Autodesk Inventor part; units mm, degrees
ref_plane "YZ Plane" through (0, 0, 0) normal (1, 0, 0) x (0, 1, 0)
ref_plane "XZ Plane" through (0, 0, 0) normal (0, 1, 0) x (-1, 0, 0)
ref_plane "XY Plane" through (0, 0, 0) normal (0, 0, 1) x (1, 0, 0)
sketch "Boceto1" plane through (0, 0, 0) normal (0, 0, 1) x (1, 0, 0)
  line L0 (0, 0) -> (11.3785, 0)
  line L1 (0, 5) -> (10, 5)
  line L2 (10, 5) -> (10, 14)
  line L3 (10, 14) -> (5, 14)
  line L4 (5, 14) -> (5, 7.5)
  line L5 (5, 7.5) -> (0, 7.5)
  line L6 (0, 7.5) -> (0, 5)
  dimension "d0" = 5
  dimension "d1" = 5
  dimension "d3" = 28
  dimension "d4" = 15
  dimension "d5" = 10
revolve "Revolución1" add sketch "Boceto1" angle 360 about axis through (0, 0, 0) along (1, 0, 0)
fillet "Empalme1" radius 1 1 edges at (5, -7.5, 0)
chamfer "Chaflán1" distance 1 angle 45 1 edges at (5, -14, 0)
sketch "Boceto2" plane through (10, 0, 0) normal (1, 0, 0) x (0, 0, -1)
  circle A0 centre (0, 0) radius 14
  line L0 (-12, 12) -> (12, 12)
  line L1 (12, 12) -> (12, -12)
  line L2 (12, -12) -> (-12, -12)
  line L3 (-12, -12) -> (-12, 12)
  point P0 (12, 0)
  point P1 (0, 12)
  point P2 (-7.2111, 12)
  point P3 (7.2111, 12)
  point P4 (12, 7.2111)
  point P5 (12, -7.2111)
  point P6 (-12, -7.2111)
  point P7 (-12, 7.2111)
  point P8 (7.2111, -12)
  point P9 (-7.2111, -12)
  dimension "d11" = 24
  dimension "d12" = 24
extrude "Extrusión1" cut sketch "Boceto2" against normal blind 2.5 contours A0 L1 | L0 A0 | A0 L2 | L3 A0
thread "Rosca1"
properties part number "tuerca_manzana_1"
Can you work these out from the model? Positions are in its coordinate system, mm. A direction names the side the tool comes from. Coordinates: 2 decimals unless noted, no trailing zeros. Loops run counter-clockwise (first coordinate to the right, second up) from the corner with the lowest first, then second, coordinate; pieces in that order, holes last. Notation, with made-up numbers: (28.25, 31.25) -> (39.25, 31.25) arc R30 ccw to (39.25, 58.25) -> close; hole circle Ø2 at (12.25, -12.75). An arc over 180 degrees is marked (long way). Answer as a JSON object with one key per item and string values.
1) Imagine slicing it at D-D (x = 1.5). Please give me the cut outline in (y, z).
Results:
{"outline": "circle Ø15 at (0, 0); hole circle Ø10 at (0, 0)"}
2) Imagine slicing it at A-A (y = 0). Please give me the cut outline in (x, z), then the cut area to 3 significant figures.
Results:
{"outline": "(0, -7.5) -> (4, -7.5) arc R1 cw to (5, -8.5) -> (5, -13) -> (6, -14) -> (7.5, -14) -> (7.5, -12) -> (10, -12) -> (10, -5) -> (0, -5) -> close; (0, 5) -> (10, 5) -> (10, 12) -> (7.5, 12) -> (7.5, 14) -> (6, 14) -> (5, 13) -> (5, 8.5) arc R1 cw to (4, 7.5) -> (0, 7.5) -> close", "area": "104 mm^2"}
3) Imagine slicing it at C-C (x = 8.25). Please give me the cut outline in (y, z).
Results:
{"outline": "(-12, -7.21) arc R14 ccw to (-7.21, -12) -> (7.21, -12) arc R14 ccw to (12, -7.21) -> (12, 7.21) arc R14 ccw to (7.21, 12) -> (-7.21, 12) arc R14 ccw to (-12, 7.21) -> close; hole circle Ø10 at (0, 0)"}
4) For faces 1 (the face through (9, 12, 0)), 2 (the face through (9, -12, 0)), 3 (the face through (1.972, -7.493, -0.33)), which set-ups out of +Z, -Z, +X, -X, +Y, -Y let a thin tool reach every point of the face, with its end or its side?
Results:
{"face 1": "+Z, -Z, +X, +Y", "face 2": "+Z, -Z, +X, -Y", "face 3": "-X"}
5) If I drill on line 1 (Z direction, x = 6.75, y = 0); line 2 (Z direction, x = 2, y = 0); line 3 (X direction, y = 5.75, z = -10), over which ranges is the centre line in solid material (lowest first)?
Results:
{"line 1": "z = -14 to -5, 5 to 14", "line 2": "z = -7.5 to -5, 5 to 7.5", "line 3": "x = 5 to 10"}
6) For P1, Ø5, axis at x = 3.5, y = 2.5, coming from the +Z side; P2, Ø3, axis at x = 9.5, y = -0.5, coming from the +Z side; P3, Ø2, axis at y = 13.5, z = -1.5, coming from the +X side; P4, Ø3, axis at y = 2.5, z = 0.5, coming from the -X side, each with a flat end and sliding along its axis, tell me the tip position at first contact or that it passes through.
Results:
{"P1": "stops at z = 13.81", "P2": "stops at z = 12", "P3": "stops at x = 7.5", "P4": "passes through"}
7) Thinking about a two-plate mould opening in Y: for faces 4 (the face through (5.07, -1.08, -4.88)), 5 (the face through (7.5, -13, 0)), 6 (the face through (7.53, -10.32, -9.46)), which applies, pulls with the +Y half, pulls with the -Y half, needs draft (parallel to the pull), parting line crosses it, or undercut?
Results:
{"face 4": "undercut", "face 5": "needs draft", "face 6": "parting line crosses it"}
